Check sheet for the modelled part. Datum: model origin and axes. Units: mm. A direction names the side the tool comes from. Give positions to 0.01 mm unless a question says otherwise; leave off trailing zeros. Loops run counter-clockwise (first coordinate to the right, second up) from the corner with the lowest first, then second, coordinate; pieces in that order, holes last. Notation, with made-up numbers: (34.5, -23) - (77.5, -23) arc R18 cw to (77.5, 1) - close; hole circle Ø11 at (67.5, 68.25). An arc over 180 degrees is marked (long way). Answer in a Markdown table with one row per item. Add a question column.
(1) Sectioned sample at C-C on x = 1900. Enter the section's corners in (y, z), then the cut area to 3 significant figures.
(2) Set-up check for faces 1 (the face through (1850.05, 1397.8, -98.6)), 2 (the face through (987, 1500, 138)): record each of +Z, -Z, +X, -X, +Y, -Y from which the full face is reachable in a straight line by a thin tool's end or side.
(3) Sectioned sample at D-D on y = 1400. Enter the section's corners in (x, z).
(4) Draft check along Y on faces 3 (the face through (123.07, 1444.36, -98.6)), 4 (the face through (1984.964, 14.258, 141.96)), 5 (the face through (0, 740, 138)), 6 (the face through (1985.742, 1484.964, 141.96)). Enter one of: released by +Y, released by -Y, zero draft, split by the parting line, or undercut.
(5) Go/stop test with a flat-tipped pin: P1, Ø1.5, axis at x = 1448, y = 249, coming from the -Z side. Record where the tip stops, or that it passes through.
(6) Sectioned sample at A-A on z = -93. Enter the section's corners in (x, y), then the cut area to 3 significant figures.
(7) Sectioned sample at B-B on y = 308.5. Enter the section's corners in (x, z).
(8) Thickness scan on L1, parallel to Z at x = 220, y = 927; L2, parallel to X at y = 1421, z = -61. Record the ranges inside material, lowest first.
from build123d import *

# Parameters (mm, degrees)
F0_W     = 2000
F0_H     = 1500
F1_DEPTH = 300
F2_R     = 50
F3_R     = 20
F4_R     = 50
F5_DEPTH = 200


with BuildPart() as f1:
    # F0 (on Top) → F1 (new body)
    with BuildSketch(Plane.XY):
        with Locations((1000, 750)):
            Rectangle(F0_W, F0_H)
    extrude(amount=F1_DEPTH)

    # F2
    f2_edges = [f1.edges().sort_by_distance(p)[0] for p in [
        (2000, 0, 150),
        (2000, 1500, 150),
        (0, 0, 150),
        (0, 1500, 150),
    ]]
    fillet(f2_edges, radius=F2_R)

    # F3
    f3_edges = [f1.edges().sort_by_distance(p)[0] for p in [
        (0, 750, 300),
        (14.644661, 1485.355339, 300),
        (14.644661, 14.644661, 300),
        (1000, 1500, 300),
        (1000, 0, 300),
        (1985.355339, 1485.355339, 300),
        (1985.355339, 14.644661, 300),
        (2000, 750, 300),
    ]]
    fillet(f3_edges, radius=F3_R)

    # F4 (on face) → F5 (join)
    with BuildSketch(Plane(origin=(0, 0, 0), x_dir=(1, 0, 0), z_dir=(0, 0, -1))):
        with Locations((100, -100)):
            Circle(F4_R)
        with Locations((100, -1400)):
            Circle(F4_R)
        with Locations((1900, -100)):
            Circle(F4_R)
        with Locations((1900, -1400)):
            Circle(F4_R)
    extrude(amount=F5_DEPTH)


solid = f1.part
Reply:
| question | item | result |
|---|---|---|
| 1 | outline | (0, 0) - (50, 0) - (50, -200) - (150, -200) - (150, 0) - (1350, 0) - (1350, -200) - (1450, -200) - (1450, 0) - (1500, 0) - (1500, 280) arc R20 ccw to (1480, 300) - (20, 300) arc R20 ccw to (0, 280) - close |
| 1 | area | 490,000 mm^2 |
| 2 | face 1 | -Z |
| 2 | face 2 | +Z, -Z, +X, -X, +Y |
| 3 | outline | (0, 0) - (50, 0) - (50, -200) - (150, -200) - (150, 0) - (1850, 0) - (1850, -200) - (1950, -200) - (1950, 0) - (2000, 0) - (2000, 280) arc R20 ccw to (1980, 300) - (20, 300) arc R20 ccw to (0, 280) - close |
| 4 | face 3 | undercut |
| 4 | face 4 | released by -Y |
| 4 | face 5 | zero draft |
| 4 | face 6 | released by +Y |
| 5 | P1 | z = 0 |
| 6 | outline | circle Ø100 at (100, 100); circle Ø100 at (100, 1400); circle Ø100 at (1900, 100); circle Ø100 at (1900, 1400) |
| 6 | area | 31,400 mm^2 |
| 7 | outline | (0, 0) - (2000, 0) - (2000, 280) arc R20 ccw to (1980, 300) - (20, 300) arc R20 ccw to (0, 280) - close |
| 8 | L1 | 0 to 300 |
| 8 | L2 | 54.62 to 145.38, 1854.62 to 1945.38 |
